For this review, use the dimensioned drawing (mm, ordinates from the lowest corner) and the shaded views. A direction names the side the tool comes from. Coordinates: 2 decimals unless noted, no trailing zeros. Order: outer loops, then holes, each group sorted by start corner. A loop starts at its lowest first (then second) coordinate and runs counter-clockwise, first axis right, second up. Notation, with made-up numbers: (48.5, -28) -> (80.5, -28) arc R22 ccw to (80.5, -9) -> close; hole circle Ø1 at (-24, 2.5). An arc over 180 degrees is marked (long way). Use one line per item in the form item = value. Start each with the question number.
(1) Take a section at C-C (z = 27.5). State the section outline as (x, y) points.
(2) Take a section at A-A (x = 66.5). State the section outline as (y, z) points.
(3) Wall thickness on line 1 along Y through (x, z) = (48.5, 28); line 2 along Z through (x, y) = (121, 14.5): over which ranges is each line inside the solid? List them lowest first.
(4) Take a section at B-B (y = 18). State the section outline as (x, z) points.
(5) For the marked faces 1 and 2, list the 3-axis set-ups (+Z, -Z, +X, -X, +Y, -Y) from which the entire face can be reached by the end or side of a thin tool; tool diameter is ignored.
(6) Insertion check: pin 1 Ø10 at (x, z) = (77.5, 19) entering from -Y; pin 2 Ø13 at (x, y) = (92, 10) entering from +Z; pin 3 Ø6 at (x, z) = (71.5, 40.5) entering from -Y. Each pin has a flat end and moves straight along its axis. Give the tip position at first contact, or say it passes through.
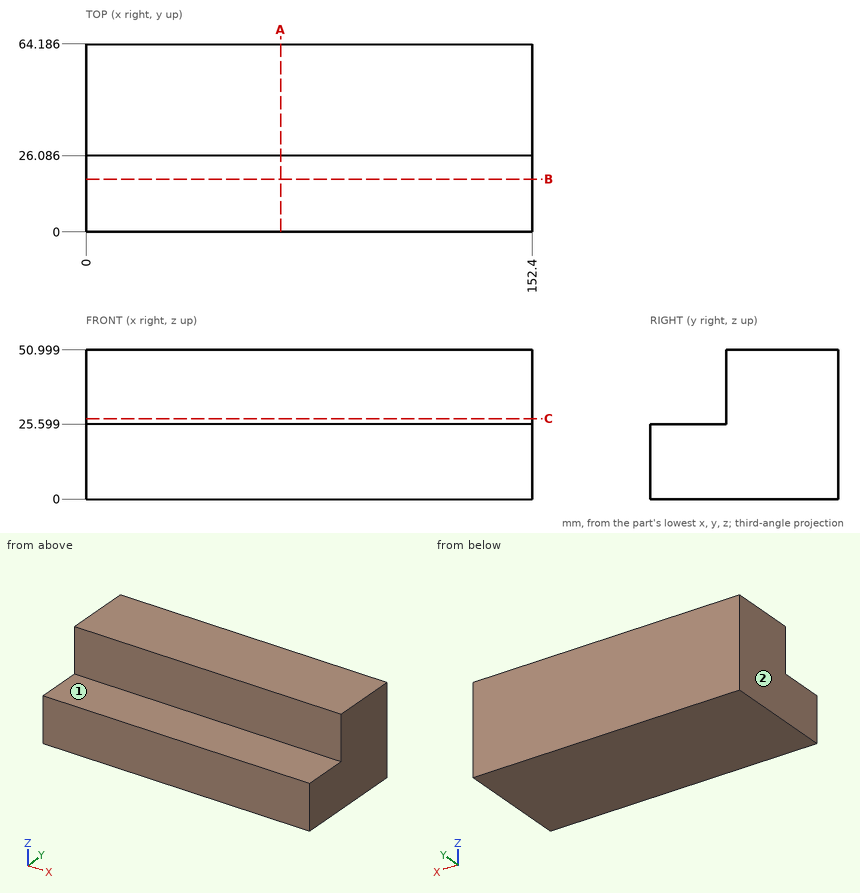
Findings:
q1.outline = (0, 26.09) -> (152.4, 26.09) -> (152.4, 64.19) -> (0, 64.19) -> close
q2.outline = (0, 0) -> (64.19, 0) -> (64.19, 51) -> (26.09, 51) -> (26.09, 25.6) -> (0, 25.6) -> close
q3.line_1 = 26.09 to 64.19
q3.line_2 = 0 to 25.6
q4.outline = (0, 0) -> (152.4, 0) -> (152.4, 25.6) -> (0, 25.6) -> close
q5.face_1 = +Z, +X, -X, -Y
q5.face_2 = +Z, -Z, -X, +Y, -Y
q6.pin_1 = 0
q6.pin_2 = 25.6
q6.pin_3 = 26.09
